The listing builds one solid part. Answer for the finished solid, in the listing's coordinates (mm). Round coordinates to 2 decimals unless told otherwise and drop trailing zeros. One line per item, written item: value.
```python
from build123d import *

# Parameters (mm, degrees)
SKETCH1_W           = 191
SKETCH1_H           = 191
SKETCH1_R           = 3
BOSS_EXTRUDE1_DEPTH = 10


with BuildPart() as part:
    # Sketch1 → Boss-Extrude1 (new body)
    with BuildSketch(Plane(origin=(0, 0, 0), x_dir=(1, 0, 0), z_dir=(0, 1, 0))):
        with Locations((95.5, 95.5)):
            Rectangle(SKETCH1_W, SKETCH1_H)
        with Locations(Location((28, 163, 0), (0, 0, 270))):
            Circle(SKETCH1_R, mode=Mode.SUBTRACT)
        with Locations(Location((48, 163, 0), (0, 0, 270))):
            Circle(SKETCH1_R, mode=Mode.SUBTRACT)
        with Locations(Location((68, 163, 0), (0, 0, 270))):
            Circle(SKETCH1_R, mode=Mode.SUBTRACT)
        with Locations(Location((88, 163, 0), (0, 0, 270))):
            Circle(SKETCH1_R, mode=Mode.SUBTRACT)
        with Locations(Location((108, 163, 0), (0, 0, 270))):
            Circle(SKETCH1_R, mode=Mode.SUBTRACT)
        with Locations(Location((48, 143, 0), (0, 0, 270))):
            Circle(SKETCH1_R, mode=Mode.SUBTRACT)
        with Locations(Location((68, 143, 0), (0, 0, 270))):
            Circle(SKETCH1_R, mode=Mode.SUBTRACT)
        with Locations(Location((88, 143, 0), (0, 0, 270))):
            Circle(SKETCH1_R, mode=Mode.SUBTRACT)
        with Locations(Location((108, 143, 0), (0, 0, 270))):
            Circle(SKETCH1_R, mode=Mode.SUBTRACT)
        with Locations(Location((48, 123, 0), (0, 0, 270))):
            Circle(SKETCH1_R, mode=Mode.SUBTRACT)
        with Locations(Location((68, 123, 0), (0, 0, 270))):
            Circle(SKETCH1_R, mode=Mode.SUBTRACT)
        with Locations(Location((88, 123, 0), (0, 0, 270))):
            Circle(SKETCH1_R, mode=Mode.SUBTRACT)
        with Locations(Location((108, 123, 0), (0, 0, 270))):
            Circle(SKETCH1_R, mode=Mode.SUBTRACT)
        with Locations(Location((48, 103, 0), (0, 0, 270))):
            Circle(SKETCH1_R, mode=Mode.SUBTRACT)
        with Locations(Location((68, 103, 0), (0, 0, 270))):
            Circle(SKETCH1_R, mode=Mode.SUBTRACT)
        with Locations(Location((88, 103, 0), (0, 0, 270))):
            Circle(SKETCH1_R, mode=Mode.SUBTRACT)
        with Locations(Location((108, 103, 0), (0, 0, 270))):
            Circle(SKETCH1_R, mode=Mode.SUBTRACT)
        with Locations(Location((48, 83, 0), (0, 0, 270))):
            Circle(SKETCH1_R, mode=Mode.SUBTRACT)
        with Locations(Location((68, 83, 0), (0, 0, 270))):
            Circle(SKETCH1_R, mode=Mode.SUBTRACT)
        with Locations(Location((88, 83, 0), (0, 0, 270))):
            Circle(SKETCH1_R, mode=Mode.SUBTRACT)
        with Locations(Location((108, 83, 0), (0, 0, 270))):
            Circle(SKETCH1_R, mode=Mode.SUBTRACT)
        with Locations(Location((28, 143, 0), (0, 0, 270))):
            Circle(SKETCH1_R, mode=Mode.SUBTRACT)
        with Locations(Location((28, 123, 0), (0, 0, 270))):
            Circle(SKETCH1_R, mode=Mode.SUBTRACT)
        with Locations(Location((28, 103, 0), (0, 0, 270))):
            Circle(SKETCH1_R, mode=Mode.SUBTRACT)
        with Locations(Location((28, 83, 0), (0, 0, 270))):
            Circle(SKETCH1_R, mode=Mode.SUBTRACT)
        with Locations(Location((28, 63, 0), (0, 0, 270))):
            Circle(SKETCH1_R, mode=Mode.SUBTRACT)
        with Locations(Location((48, 63, 0), (0, 0, 270))):
            Circle(SKETCH1_R, mode=Mode.SUBTRACT)
        with Locations(Location((68, 63, 0), (0, 0, 270))):
            Circle(SKETCH1_R, mode=Mode.SUBTRACT)
        with Locations(Location((88, 63, 0), (0, 0, 270))):
            Circle(SKETCH1_R, mode=Mode.SUBTRACT)
        with Locations(Location((108, 63, 0), (0, 0, 270))):
            Circle(SKETCH1_R, mode=Mode.SUBTRACT)
        with Locations(Location((28, 43, 0), (0, 0, 270))):
            Circle(SKETCH1_R, mode=Mode.SUBTRACT)
        with Locations(Location((48, 43, 0), (0, 0, 270))):
            Circle(SKETCH1_R, mode=Mode.SUBTRACT)
        with Locations(Location((68, 43, 0), (0, 0, 270))):
            Circle(SKETCH1_R, mode=Mode.SUBTRACT)
        with Locations(Location((88, 43, 0), (0, 0, 270))):
            Circle(SKETCH1_R, mode=Mode.SUBTRACT)
        with Locations(Location((108, 43, 0), (0, 0, 270))):
            Circle(SKETCH1_R, mode=Mode.SUBTRACT)
        with Locations(Location((28, 23, 0), (0, 0, 270))):
            Circle(SKETCH1_R, mode=Mode.SUBTRACT)
        with Locations(Location((48, 23, 0), (0, 0, 270))):
            Circle(SKETCH1_R, mode=Mode.SUBTRACT)
        with Locations(Location((68, 23, 0), (0, 0, 270))):
            Circle(SKETCH1_R, mode=Mode.SUBTRACT)
        with Locations(Location((88, 23, 0), (0, 0, 270))):
            Circle(SKETCH1_R, mode=Mode.SUBTRACT)
        with Locations(Location((108, 23, 0), (0, 0, 270))):
            Circle(SKETCH1_R, mode=Mode.SUBTRACT)
        with Locations(Location((128, 163, 0), (0, 0, 270))):
            Circle(SKETCH1_R, mode=Mode.SUBTRACT)
        with Locations(Location((148, 163, 0), (0, 0, 270))):
            Circle(SKETCH1_R, mode=Mode.SUBTRACT)
        with Locations(Location((168, 163, 0), (0, 0, 270))):
            Circle(SKETCH1_R, mode=Mode.SUBTRACT)
        with Locations(Location((128, 143, 0), (0, 0, 270))):
            Circle(SKETCH1_R, mode=Mode.SUBTRACT)
        with Locations(Location((148, 143, 0), (0, 0, 270))):
            Circle(SKETCH1_R, mode=Mode.SUBTRACT)
        with Locations(Location((168, 143, 0), (0, 0, 270))):
            Circle(SKETCH1_R, mode=Mode.SUBTRACT)
        with Locations(Location((128, 123, 0), (0, 0, 270))):
            Circle(SKETCH1_R, mode=Mode.SUBTRACT)
        with Locations(Location((148, 123, 0), (0, 0, 270))):
            Circle(SKETCH1_R, mode=Mode.SUBTRACT)
        with Locations(Location((168, 123, 0), (0, 0, 270))):
            Circle(SKETCH1_R, mode=Mode.SUBTRACT)
        with Locations(Location((128, 103, 0), (0, 0, 270))):
            Circle(SKETCH1_R, mode=Mode.SUBTRACT)
        with Locations(Location((148, 103, 0), (0, 0, 270))):
            Circle(SKETCH1_R, mode=Mode.SUBTRACT)
        with Locations(Location((168, 103, 0), (0, 0, 270))):
            Circle(SKETCH1_R, mode=Mode.SUBTRACT)
        with Locations(Location((128, 83, 0), (0, 0, 270))):
            Circle(SKETCH1_R, mode=Mode.SUBTRACT)
        with Locations(Location((148, 83, 0), (0, 0, 270))):
            Circle(SKETCH1_R, mode=Mode.SUBTRACT)
        with Locations(Location((168, 83, 0), (0, 0, 270))):
            Circle(SKETCH1_R, mode=Mode.SUBTRACT)
        with Locations(Location((128, 63, 0), (0, 0, 270))):
            Circle(SKETCH1_R, mode=Mode.SUBTRACT)
        with Locations(Location((148, 63, 0), (0, 0, 270))):
            Circle(SKETCH1_R, mode=Mode.SUBTRACT)
        with Locations(Location((168, 63, 0), (0, 0, 270))):
            Circle(SKETCH1_R, mode=Mode.SUBTRACT)
        with Locations(Location((128, 43, 0), (0, 0, 270))):
            Circle(SKETCH1_R, mode=Mode.SUBTRACT)
        with Locations(Location((148, 43, 0), (0, 0, 270))):
            Circle(SKETCH1_R, mode=Mode.SUBTRACT)
        with Locations(Location((168, 43, 0), (0, 0, 270))):
            Circle(SKETCH1_R, mode=Mode.SUBTRACT)
        with Locations(Location((128, 23, 0), (0, 0, 270))):
            Circle(SKETCH1_R, mode=Mode.SUBTRACT)
        with Locations(Location((148, 23, 0), (0, 0, 270))):
            Circle(SKETCH1_R, mode=Mode.SUBTRACT)
        with Locations(Location((168, 23, 0), (0, 0, 270))):
            Circle(SKETCH1_R, mode=Mode.SUBTRACT)
    extrude(amount=BOSS_EXTRUDE1_DEPTH)


solid = part.part
```
1) This flat-tipped pin is pushed along its axis until it touches: pin 1 Ø5 at (x, z) = (128, -63) entering from -Y. Where does it stop, or does it pass through?
Final values:
pin 1: through
2) For a pull along Z with two mould halves and no side action, classify faces 1 (the flat face through (0, 5, -94)), 2 (the cylindrical face through (106.2, 4.9, -65.4)) as released by +Z, released by -Z, zero draft, split by the parting line, or undercut.
Final values:
face 1: zero draft
face 2: undercut
3) A cutting plane is placed at A-A on x = 68. Give the number of separate pieces and of enclosed holes in the cut face, and give its area (3 significant figures).
Final values:
separate pieces: 9
enclosed holes: 0
area: 1,430 mm2
